Work out the finished part from the listing and answer in its coordinate system (mm). Coordinates: 2 decimals unless noted, no trailing zeros. Write each loop counter-clockwise with the first axis right and the second up, starting at its lowest first coordinate (ties: lowest second). Pieces come first, ordered by that corner, then holes. Notation, with made-up numbers: (-17.75, -11.5) - (-0.75, -11.5) arc R25 ccw to (-0.75, 11.5) - close; hole circle Ø9 at (-19, 0). An arc over 180 degrees is marked (long way). One line per item, written item: value.
```python
from build123d import *

# Parameters (mm, degrees)
SKETCH1_R           = 2.1
BOSS_EXTRUDE1_DEPTH = 1.5


with BuildPart() as part:
    # Sketch1 → Boss-Extrude1 (new, symmetric)
    with BuildSketch(Plane(origin=(0, 0, 0), x_dir=(1, 0, 0), z_dir=(0, 1, 0))):
        with BuildLine():
            Line((-50, 5), (50, 5))
            ThreePointArc((50, 5), (55, 0), (50, -5))
            Line((50, -5), (-50, -5))
            ThreePointArc((-50, -5), (-55, 0), (-50, 5))
        make_face()
        with Locations(Location((50, 0, 0), (0, 0, 270))):
            Circle(SKETCH1_R, mode=Mode.SUBTRACT)
        with Locations(Location((40, 0, 0), (0, 0, 270))):
            Circle(SKETCH1_R, mode=Mode.SUBTRACT)
        with Locations(Location((30, 0, 0), (0, 0, 270))):
            Circle(SKETCH1_R, mode=Mode.SUBTRACT)
        with Locations(Location((20, 0, 0), (0, 0, 270))):
            Circle(SKETCH1_R, mode=Mode.SUBTRACT)
        with Locations(Location((10, 0, 0), (0, 0, 270))):
            Circle(SKETCH1_R, mode=Mode.SUBTRACT)
        with Locations(Location((0, 0, 0), (0, 0, 270))):
            Circle(SKETCH1_R, mode=Mode.SUBTRACT)
        with Locations(Location((-10, 0, 0), (0, 0, 270))):
            Circle(SKETCH1_R, mode=Mode.SUBTRACT)
        with Locations(Location((-20, 0, 0), (0, 0, 270))):
            Circle(SKETCH1_R, mode=Mode.SUBTRACT)
        with Locations(Location((-30, 0, 0), (0, 0, 270))):
            Circle(SKETCH1_R, mode=Mode.SUBTRACT)
        with Locations(Location((-40, 0, 0), (0, 0, 270))):
            Circle(SKETCH1_R, mode=Mode.SUBTRACT)
        with Locations(Location((-50, 0, 0), (0, 0, 270))):
            Circle(SKETCH1_R, mode=Mode.SUBTRACT)
    extrude(amount=BOSS_EXTRUDE1_DEPTH, both=True)


solid = part.part
```
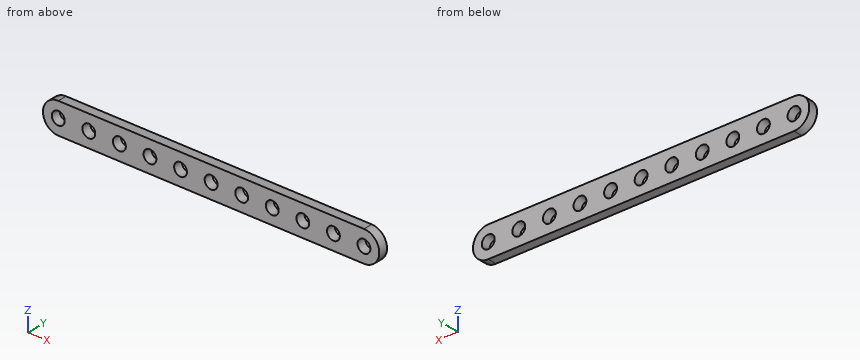
Item 1: Section C-C, the plane z = 4 is taken. Determine the outline of the cut face in (x, y).
Evaluation:
outline: (-53, -1.5) - (53, -1.5) - (53, 1.5) - (-53, 1.5) - close
Item 2: Section A-A, the plane x = 10 is taken. Determine the outline of the cut face in (y, z).
Evaluation:
outline: (-1.5, -5) - (1.5, -5) - (1.5, -2.1) - (-1.5, -2.1) - close; (-1.5, 2.1) - (1.5, 2.1) - (1.5, 5) - (-1.5, 5) - close
Item 3: Given pin 1 (5.5 mm diameter, centred on x = 20, z = 0, fed in from +Y); pin 2 (1 mm diameter, centred on y = -0.5, z = -1.5, fed in from +X), each flat-ended and moving along its own axis, determine where each tip first touches the part or whether it passes through.
Evaluation:
pin 1: stops at y = 1.5
pin 2: stops at x = 54.9
Item 4: Consider probe 1 along Z at (x, y) = (-31, 0.3); probe 2 along X at (y, z) = (-0.2, -4.5); probe 3 along X at (y, z) = (1.1, 3). Determine where each line is inside the solid, lowest interval first.
Evaluation:
probe 1: z = -5 to -1.85, 1.85 to 5
probe 2: x = -52.18 to 52.18
probe 3: x = -54 to 54
Item 5: Section B-B, the plane y = -0.05 is taken. Give the number of separate pieces and of enclosed holes in the cut face, then the cut area to 3 significant figures.
Evaluation:
separate pieces: 1
enclosed holes: 11
area: 926 mm2
